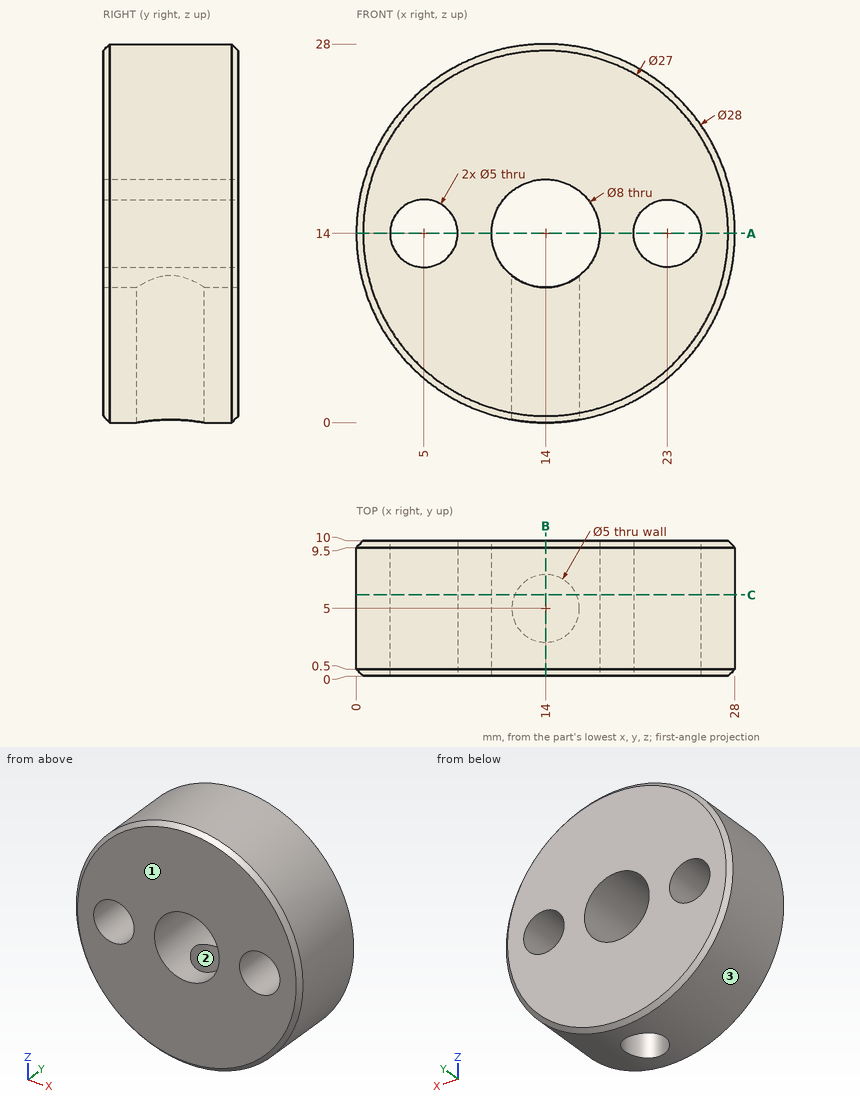
Could you check a few things on this drawing? It's one solid part, dimensions in mm from its lowest x, y, z. Give positions to 0.01 mm unless a question says otherwise; leave off trailing zeros. Order: outer loops, then holes, each group sorted by start corner. A loop starts at its lowest first (then second) coordinate and runs counter-clockwise, first axis right, second up. Notation, with made-up numbers: (15.5, -25.5) -> (69.5, -25.5) arc R4 cw to (69.5, -19.5) -> close; hole circle Ø6 at (-10.5, -19.5). An arc over 180 degrees is marked (long way). Use CSV: the item, a comma, the result in double quotes. Start each with the question number.
Item 1: Thinking about a two-plate mould opening in X: for the marked faces 1, 2 and 3, which applies, pulls with the +X half, pulls with the -X half, needs draft (parallel to the pull), parting line crosses it, or undercut?
Item 2: Suppose I cut it at B-B (x = 14). List the corners of the cut face in (y, z) for me, and give its area (4 significant figures).
Item 3: If I drill on probe 1 along Y at (x, z) = (14, 6.5); probe 2 along X at (y, z) = (8, 12.25); probe 3 along Z at (x, y) = (20.75, 4.75), over which ranges is the centre line in solid material (lowest first)? Write a range as [from, to].
Item 4: Suppose I cut it at C-C (y = 6). List the corners of the cut face in (x, z) for me, and give its area (3 significant figures).
Item 5: I'm going to push flat-ended pins straight in: P1, Ø8, axis at x = 5, z = 14, coming from the +Y side; P2, Ø4.5, axis at x = 14, y = 5, coming from the -Z side. Where does each tip first touch, or does it pass through?
Item 6: Suppose I cut it at A-A (z = 14). List the corners of the cut face in (x, y) for me, and give its area (3 significant figures).
Answer block:
1,face 1,"needs draft"
1,face 2,"undercut"
1,face 3,"parting line crosses it"
2,outline,"(0, 0.5) -> (0.5, 0) -> (2.5, 0) -> (2.5, 10) -> (0, 10) -> close; (0, 18) -> (10, 18) -> (10, 27.5) -> (9.5, 28) -> (0.5, 28) -> (0, 27.5) -> close; (7.5, 0) -> (9.5, 0) -> (10, 0.5) -> (10, 10) -> (7.5, 10) -> close"
2,area,"149.5 mm^2"
3,probe 1,"y = [0, 2.5], [7.5, 10]"
3,probe 2,"x = [0.11, 3.21], [6.79, 10.4], [17.6, 21.21], [24.79, 27.89]"
3,probe 3,"z = [1.73, 12.91], [15.09, 26.27]"
4,outline,"(11.71, 0.19) -> (11.71, 10.72) arc R4 cw (long way) to (16.29, 10.72) -> (16.29, 0.19) arc R14 ccw (long way) to start; hole circle Ø5 at (5, 14); hole circle Ø5 at (23, 14)"
4,area,"480 mm^2"
5,P1,"stops at y = 10"
5,P2,"stops at z = 17.31"
6,outline,"(0, 0.5) -> (0.5, 0) -> (2.5, 0) -> (2.5, 10) -> (0.5, 10) -> (0, 9.5) -> close; (7.5, 0) -> (10, 0) -> (10, 10) -> (7.5, 10) -> close; (18, 0) -> (20.5, 0) -> (20.5, 10) -> (18, 10) -> close; (25.5, 0) -> (27.5, 0) -> (28, 0.5) -> (28, 9.5) -> (27.5, 10) -> (25.5, 10) -> close"
6,area,"99.5 mm^2"
